Source: three-view drawing plus pictorial views. Frame: mm from the lowest corner of the part. A direction names the side the tool comes from. Give positions to 0.01 mm unless a question says otherwise; leave off trailing zeros. Order: outer loops, then holes, each group sorted by start corner. A loop starts at its lowest first (then second) coordinate and runs counter-clockwise, first axis right, second up. Notation, with made-up numbers: (46, -2) -> (82, -2) arc R13 ccw to (82, 15) -> close; hole circle Ø8 at (-0.5, 67). An arc over 180 degrees is marked (long way). Write item = value, one per line.
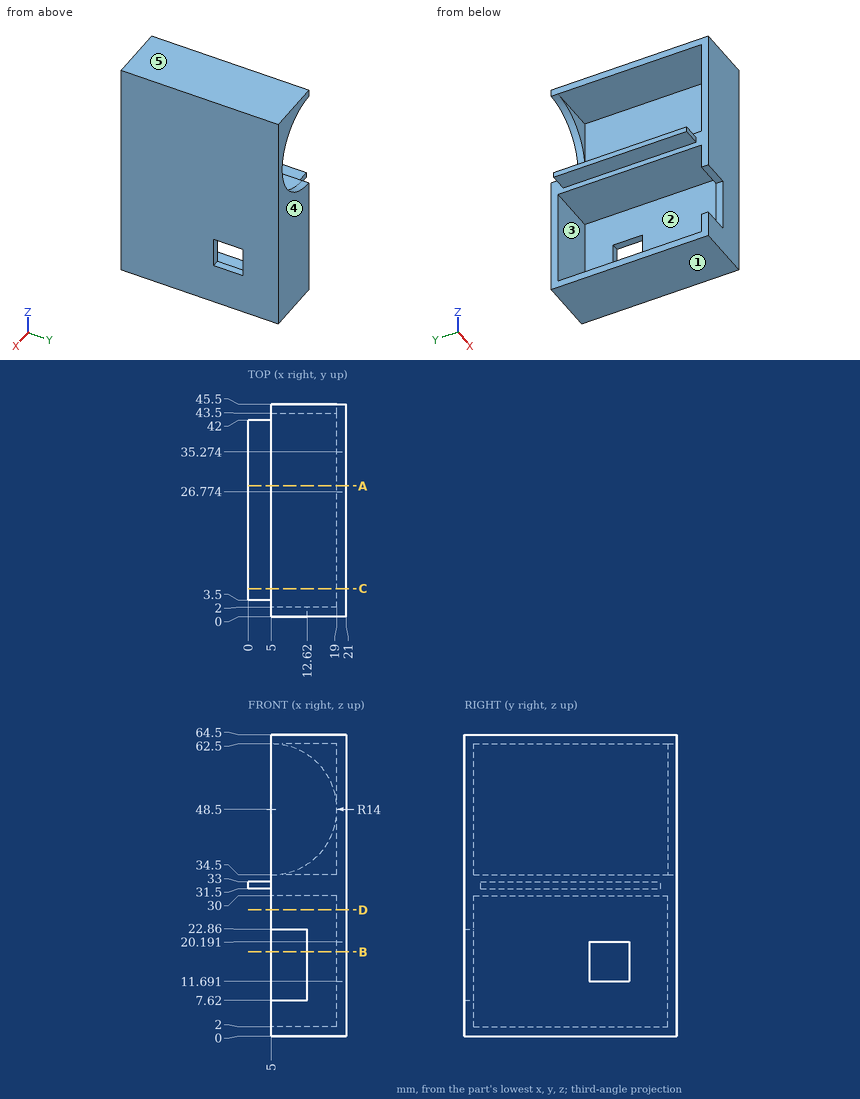
1) Reachability of the marked faces 1 and 2 from +Z, -Z, +X, -X, +Y, -Y: full face, straight path, thin tool, end or side. Return the list, or none.
Check sheet entries:
face_1 = -Z, +X, -X, +Y, -Y
face_2 = -X
2) First-contact query: P1, Ø4, axis at x = 13, z = 51, coming from the +Y side; P2, Ø4, axis at x = 10.5, z = 14.5, coming from the -Y side; P3, Ø1.6, axis at y = 1, z = 12.5, coming from the -X side. Flat tips, straight axial feed; report the tip coordinate or a pass-through.
Check sheet entries:
P1 = 2
P2 = 43.5
P3 = 12.62
3) Mould query, pull axis Y, two halves, no side actions, for the marked faces 3, 4 and 5. Classes: +Y half, -Y half, draft (parallel to the pull), parting line (faces both ways), or undercut.
Check sheet entries:
face_3 = undercut
face_4 = +Y half
face_5 = draft
4) Section query A-A (y = 28). Output: boundary loops of the cut face in (x, z), plus the area to 4 significant figures.
Check sheet entries:
outline = (0, 31.5) -> (5, 31.5) -> (5, 30) -> (19, 30) -> (19, 20.19) -> (21, 20.19) -> (21, 64.5) -> (5, 64.5) -> (5, 62.5) -> (19, 62.5) -> (19, 34.5) -> (5, 34.5) -> (5, 33) -> (0, 33) -> close; (5, 0) -> (21, 0) -> (21, 11.69) -> (19, 11.69) -> (19, 2) -> (5, 2) -> close
area = 238.5 mm²
5) Section query B-B (z = 18). Output: boundary loops of the cut face in (x, y).
Check sheet entries:
outline = (5, 43.5) -> (19, 43.5) -> (19, 35.27) -> (21, 35.27) -> (21, 45.5) -> (5, 45.5) -> close; (12.62, 0) -> (21, 0) -> (21, 26.77) -> (19, 26.77) -> (19, 2) -> (12.62, 2) -> close
6) Section query D-D (z = 27). Output: boundary loops of the cut face in (x, y), plus the area to 3 significant figures.
Check sheet entries:
outline = (5, 0) -> (21, 0) -> (21, 45.5) -> (5, 45.5) -> (5, 43.5) -> (19, 43.5) -> (19, 2) -> (5, 2) -> close
area = 147 mm²
7) Line query: line 1 (Z direction, x = 18, y = 26.5); line 2 (Y direction, x = 12.75, z = 13.5); line 3 (X direction, y = 38, z = 42). Output: solid intervals per line, ascending. Write a range as from..to.
Check sheet entries:
line_1 = 0..2, 30..34.5, 62.5..64.5
line_2 = 0..2, 43.5..45.5
line_3 = 19..21
8) Section query C-C (y = 6). Output: boundary loops of the cut face in (x, z).
Check sheet entries:
outline = (0, 31.5) -> (5, 31.5) -> (5, 30) -> (19, 30) -> (19, 2) -> (5, 2) -> (5, 0) -> (21, 0) -> (21, 64.5) -> (5, 64.5) -> (5, 62.5) -> (19, 62.5) -> (19, 34.5) -> (5, 34.5) -> (5, 33) -> (0, 33) -> close
